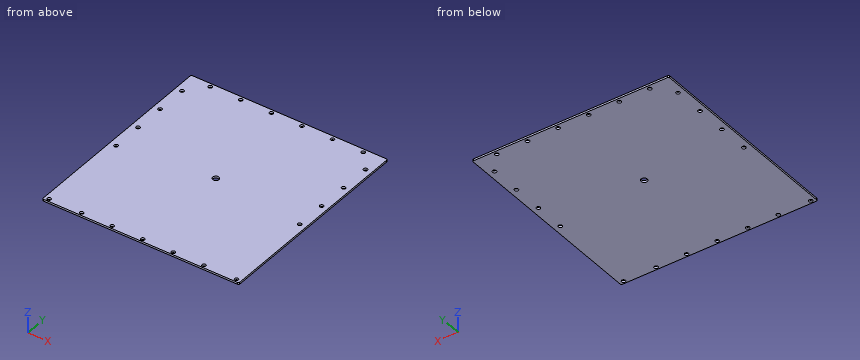
from build123d import *

# Parameters (mm, degrees)
SKETCH2_W           = 163.1
SKETCH2_H           = 171.98
SKETCH2_R           = 2.5527
SKETCH2_R_2         = 1.5875
BOSS_EXTRUDE2_DEPTH = 1.5875
FILLET1_R           = 1


with BuildPart() as part:
    # Sketch2 → Boss-Extrude2 (new body)
    with BuildSketch(Plane.XY):
        with Locations((82.55, -85.99)):
            Rectangle(SKETCH2_W, SKETCH2_H)
        with Locations((82.55, -85)):
            Circle(SKETCH2_R, mode=Mode.SUBTRACT)
        with Locations((82.55, -169.48)):
            Circle(SKETCH2_R_2, mode=Mode.SUBTRACT)
        with Locations((4.7625, -169.48)):
            Circle(SKETCH2_R_2, mode=Mode.SUBTRACT)
        with Locations((31.75, -169.48)):
            Circle(SKETCH2_R_2, mode=Mode.SUBTRACT)
        with Locations((57.15, -169.48)):
            Circle(SKETCH2_R_2, mode=Mode.SUBTRACT)
        with Locations((6.35, -94.25)):
            Circle(SKETCH2_R_2, mode=Mode.SUBTRACT)
        with Locations((6.35, -68.85)):
            Circle(SKETCH2_R_2, mode=Mode.SUBTRACT)
        with Locations((6.35, -43.45)):
            Circle(SKETCH2_R_2, mode=Mode.SUBTRACT)
        with Locations((6.35, -18.05)):
            Circle(SKETCH2_R_2, mode=Mode.SUBTRACT)
        with Locations((19.05, -3.175)):
            Circle(SKETCH2_R_2, mode=Mode.SUBTRACT)
        with Locations((44.45, -3.175)):
            Circle(SKETCH2_R_2, mode=Mode.SUBTRACT)
        with Locations((69.85, -3.175)):
            Circle(SKETCH2_R_2, mode=Mode.SUBTRACT)
        with Locations((158.75, -43.45)):
            Circle(SKETCH2_R_2, mode=Mode.SUBTRACT)
        with Locations((158.75, -18.05)):
            Circle(SKETCH2_R_2, mode=Mode.SUBTRACT)
        with Locations((146.05, -3.175)):
            Circle(SKETCH2_R_2, mode=Mode.SUBTRACT)
        with Locations((107.95, -169.48)):
            Circle(SKETCH2_R_2, mode=Mode.SUBTRACT)
        with Locations((133.35, -169.48)):
            Circle(SKETCH2_R_2, mode=Mode.SUBTRACT)
        with Locations((160.3375, -169.48)):
            Circle(SKETCH2_R_2, mode=Mode.SUBTRACT)
        with Locations((158.75, -94.25)):
            Circle(SKETCH2_R_2, mode=Mode.SUBTRACT)
        with Locations((158.75, -68.85)):
            Circle(SKETCH2_R_2, mode=Mode.SUBTRACT)
        with Locations((95.25, -3.175)):
            Circle(SKETCH2_R_2, mode=Mode.SUBTRACT)
        with Locations((120.65, -3.175)):
            Circle(SKETCH2_R_2, mode=Mode.SUBTRACT)
    extrude(amount=BOSS_EXTRUDE2_DEPTH)

    # Fillet1
    fillet1_edges = [part.edges().sort_by_distance(p)[0] for p in [
        (1, -171.98, 0.79375),
        (1, 0, 0.79375),
        (164.1, 0, 0.79375),
        (164.1, -171.98, 0.79375),
    ]]
    fillet(fillet1_edges, radius=FILLET1_R)


solid = part.part
Design review of the part built by this model. Coordinates are the model's own, in mm. Round coordinates to 2 decimals unless told otherwise and drop trailing zeros. Loops run counter-clockwise (first coordinate to the right, second up) from the corner with the lowest first, then second, coordinate; pieces in that order, holes last. Notation, with made-up numbers: (37, 2.25) - (94, 2.25) arc R20 cw to (94, 18.25) - close; hole circle Ø1 at (37.25, 45.5). An arc over 180 degrees is marked (long way). One line per question, with ' | ' between items.
1. We need section A-A, the plane y = -85. State the section outline as (x, z) points.
Results are:
outline: (1, 0) - (80, 0) - (80, 1.59) - (1, 1.59) - close; (85.1, 0) - (164.1, 0) - (164.1, 1.59) - (85.1, 1.59) - close
2. For L1, parallel to X at y = -94.25, z = 1.1; L2, parallel to Y at x = 82.5, z = 1.25; L3, parallel to X at y = -95.5, z = 0.95, list the stretches that pass through material, from the lowest coordinate up. Write a range as [from, to].
Results are:
L1: x = [1, 4.76], [7.94, 157.16], [160.34, 164.1] | L2: y = [-171.98, -171.07], [-167.89, -87.55], [-82.45, 0] | L3: x = [1, 5.37], [7.33, 157.77], [159.73, 164.1]
3. Clearance check with a flat-ended pin moving along its axis: P1, Ø1.9, axis at x = 160.34, y = -169.48, coming from the -Z side. State where the tip first meets the part, or that it passes through.
Results are:
P1: passes through
